The model under review builds one solid part; all positions refer to its coordinate system, in mm. A direction names the side the tool comes from. Coordinates: 2 decimals unless noted, no trailing zeros. Loops run counter-clockwise (first coordinate to the right, second up) from the corner with the lowest first, then second, coordinate; pieces in that order, holes last. Notation, with made-up numbers: M 18.5,58.25 L 23.5,58.25 A33 ccw 23.5,86.25 Z; hole C -30.5,83.25 d5. An arc over 180 degrees is marked long. Write item = value, one per line. Start each with the question number.
Q1. For faces 5 (the face through (-4.42, 1.54, 15)), 6 (the face through (0, 0, 0)), 7 (the face through (-0.1, -6.2, 42)), list the 3-axis set-ups (+Z, -Z, +X, -X, +Y, -Y) from which the entire face can be reached by the end or side of a thin tool; tool diameter is ignored.
Q2. We need section B-B on z = 22.5. Give the boundary of the cut face in (x, y), and give its area (3 significant figures).
Q3. Wall thickness on probe 1 along Z at (x, y) = (1, 6); probe 2 along Z at (x, y) = (-2.25, 6.25); probe 3 along Z at (x, y) = (2.5, -0.25): over which ranges is each line inside the solid? List them lowest first.
Q4. Clearance check with flat-ended pins moving along their axes: pin 1 Ø3 at (y, z) = (6, 23) entering from -X; pin 2 Ø6 at (x, z) = (4, 42.5) entering from +Y; pin 3 Ø1 at (y, z) = (-6.5, 37.5) entering from -X. State where each tip first meets the part, or that it passes through.
Q5. Mouldability with a two-part tool opening along Y and no side actions: class faces 1 (the face through (-4, 1, 66)), 2 (the face through (-0.469, 3.573, 65.507)), 3 (the face through (0, 0, 65)), 4 (the face through (-5.158, -3.955, 22.395)) as released by +Y, released by -Y, zero draft, split by the parting line, or undercut.
Q6. We need section C-C on z = 4.5. Give the boundary of the cut face in (x, y).
Q7. We need section A-A on z = 40.5. Give the boundary of the cut face in (x, y).
from build123d import *

# Parameters (mm, degrees)
SKETCH_1_R          = 4.5
EXTRUDE_1_DEPTH     = 15
SKETCH_2_R          = 6.5
EXTRUDE_2_DEPTH     = 15
EXTRUDE_3_DEPTH     = 12
SKETCH_4_R          = 6
EXTRUDE_4_DEPTH     = 4
SKETCH_5_RX         = 7.512684998
SKETCH_5_RY         = 6.53508396
EXTRUDE_5_DEPTH     = 20
SKETCH_6_R          = 3.603234424
CUT_EXTRUDE_1_DEPTH = 1


with BuildPart() as part:
    # ｽｹｯﾁ1 → ﾎﾞｽ - 押し出し1 (new body)
    with BuildSketch(Plane.XY):
        Circle(SKETCH_1_R)
    extrude(amount=EXTRUDE_1_DEPTH)

    # ｽｹｯﾁ2 → ﾎﾞｽ - 押し出し2 (add)
    with BuildSketch(Plane.XY.offset(15)):
        Circle(SKETCH_2_R)
    extrude(amount=EXTRUDE_2_DEPTH)

    # ｽｹｯﾁ3 → ﾎﾞｽ - 押し出し3 (add)
    with BuildSketch(Plane.XY.offset(30)):
        Polygon((0, -9.548712613), (8.269427696, -4.774356306), (8.269427696, 4.774356306), (0, 9.548712613), (-8.269427696, 4.774356306), (-8.269427696, -4.774356306), align=None)
    extrude(amount=EXTRUDE_3_DEPTH)

    # ｽｹｯﾁ4 → ﾎﾞｽ - 押し出し4 (add)
    with BuildSketch(Plane.XY.offset(42)):
        Circle(SKETCH_4_R)
    extrude(amount=EXTRUDE_4_DEPTH)

    # ｽｹｯﾁ5 → ﾎﾞｽ - 押し出し5 (add)
    with BuildSketch(Plane.XY.offset(46)):
        with Locations(Location((0, 0), (0, 0, -33.587248831))):
            Ellipse(SKETCH_5_RX, SKETCH_5_RY)
    extrude(amount=EXTRUDE_5_DEPTH)

    # ｽｹｯﾁ6 → ｶｯﾄ - 押し出し1 (cut)
    with BuildSketch(Plane.XY.offset(66)):
        Circle(SKETCH_6_R)
    extrude(amount=-CUT_EXTRUDE_1_DEPTH, mode=Mode.SUBTRACT)


solid = part.part
Returned:
q1.face_5 = -Z
q1.face_6 = -Z, +X, -X, +Y, -Y
q1.face_7 = none
q2.outline = C 0,0 d13
q2.area = 133 mm^2
q3.probe_1 = 15 to 42, 46 to 66
q3.probe_2 = 30 to 42, 46 to 66
q3.probe_3 = 0 to 65
q4.pin_1 = -4.69
q4.pin_2 = 8.95
q4.pin_3 = -6.15
q5.face_1 = zero draft
q5.face_2 = undercut
q5.face_3 = undercut
q5.face_4 = split by the parting line
q6.outline = C 0,0 d9
q7.outline = M -8.27,-4.77 L 0,-9.55 L 8.27,-4.77 L 8.27,4.77 L 0,9.55 L -8.27,4.77 Z
